from build123d import *

# Parameters (mm, degrees)
SKETCH1_R                 = 3.2639
BOSS_EXTRUDE1_DEPTH       = 12.7
SKETCH2_W                 = 12.7
SKETCH2_H                 = 12.7
CUT_EXTRUDE1_DEPTH        = 6.35
SKETCH3_W                 = 9.525
SKETCH3_H                 = 12.7
CUT_EXTRUDE2_DEPTH        = 9.525
F_6_32_TAPPED_HOLE1_D     = 2.7051
F_6_32_TAPPED_HOLE1_DEPTH = 15.875
F_6_32_TAPPED_HOLE1_TIP   = 0.81269403


with BuildPart() as part:
    # Sketch1 → Boss-Extrude1 (new body)
    with BuildSketch(Plane.XY):
        with BuildLine():
            Line((-7.9375, 13.335), (-7.9375, 38.1))
            Line((-7.9375, 38.1), (7.9375, 38.1))
            Line((7.9375, 38.1), (7.9375, 13.335))
            ThreePointArc((7.9375, 13.335), (9.983359133, 8.395859133), (14.9225, 6.35))
            Line((14.9225, 6.35), (66.294, 6.35))
            ThreePointArc((66.294, 6.35), (66.563407684, 6.238407684), (66.675, 5.969))
            Line((66.675, 5.969), (66.675, -5.969))
            ThreePointArc((66.675, -5.969), (66.563407684, -6.238407684), (66.294, -6.35))
            Line((66.294, -6.35), (-66.294, -6.35))
            ThreePointArc((-66.294, -6.35), (-66.563407684, -6.238407684), (-66.675, -5.969))
            Line((-66.675, -5.969), (-66.675, 5.969))
            ThreePointArc((-66.675, 5.969), (-66.563407684, 6.238407684), (-66.294, 6.35))
            Line((-66.294, 6.35), (-14.9225, 6.35))
            ThreePointArc((-14.9225, 6.35), (-9.983359133, 8.395859133), (-7.9375, 13.335))
        make_face()
        with Locations((-60.325, 0)):
            Circle(SKETCH1_R, mode=Mode.SUBTRACT)
        with Locations((60.325, 0)):
            Circle(SKETCH1_R, mode=Mode.SUBTRACT)
    extrude(amount=BOSS_EXTRUDE1_DEPTH)

    # Sketch2 → Cut-Extrude1 (cut)
    with BuildSketch(Plane(origin=(0, 0, 0), x_dir=(-1, 0, 0), z_dir=(0, 0, -1))):
        with Locations((-60.325, 0)):
            Rectangle(SKETCH2_W, SKETCH2_H)
        with Locations((60.325, 0)):
            Rectangle(SKETCH2_W, SKETCH2_H)
    extrude(amount=-CUT_EXTRUDE1_DEPTH, mode=Mode.SUBTRACT)

    # Sketch3 → Cut-Extrude2 (cut)
    with BuildSketch(Plane(origin=(0, 38.1, 0), x_dir=(1, 0, 0), z_dir=(0, 1, 0))):
        with Locations((0, -6.35)):
            Rectangle(SKETCH3_W, SKETCH3_H)
    extrude(amount=-CUT_EXTRUDE2_DEPTH, mode=Mode.SUBTRACT)

    # #6-32 Tapped Hole1
    with Locations(Plane(origin=(0, 28.575, 0), x_dir=(1, 0, 0), z_dir=(0, 1, 0))):
        with Locations((0, -3.175), (0, -9.525)):
            Hole(F_6_32_TAPPED_HOLE1_D / 2, depth=F_6_32_TAPPED_HOLE1_DEPTH)
            with Locations((0, 0, -(F_6_32_TAPPED_HOLE1_DEPTH + F_6_32_TAPPED_HOLE1_TIP / 2))):  # 118° drill point
                Cone(0, F_6_32_TAPPED_HOLE1_D / 2, F_6_32_TAPPED_HOLE1_TIP, mode=Mode.SUBTRACT)


solid = part.part
Verification items for the finished model (mm, model axes). A direction names the side the tool comes from. Give positions to 0.01 mm unless a question says otherwise; leave off trailing zeros. Write each loop counter-clockwise with the first axis right and the second up, starting at its lowest first coordinate (ties: lowest second). Pieces come first, ordered by that corner, then holes. Notation, with made-up numbers: M 84.25,6 L 114.25,6 A24 cw 114.25,25 Z; hole C 71.5,51.5 d11. An arc over 180 degrees is marked long. Write item = value, one per line.
(1) Draft check along X on faces 1 (the face through (-4.762, 33, 6)), 2 (the face through (-53.975, 0, 3)), 3 (the face through (9.93, 8.45, 6.26)). Enter one of: released by +X, released by -X, zero draft, split by the parting line, or undercut.
Found:
face_1 = undercut
face_2 = released by -X
face_3 = released by +X
(2) Sectioned sample at C-C (x = 3.5). Record the cut outline in (y, z) (3 decimals), then the cut area to 3 significant figures.
Found:
outline = M -6.35,0 L 28.575,0 L 28.575,12.7 L -6.35,12.7 Z
area = 444 mm2
(3) Access from +Z, -Z, +X, -X, +Y, -Y to the whole of each face (thin tool, end or side, straight path). Record for faces 4 (the face through (40, 6.35, 6)), 5 (the face through (62, 3, 6.35)), 6 (the face through (0, 28.575, 6)).
Found:
face_4 = +Z, -Z, +X, +Y
face_5 = -Z, +X, +Y, -Y
face_6 = +Z, -Z, +Y
(4) Go/stop test with flat-tipped pins: pin 1 Ø1.6 at (x, z) = (0, 9.525) entering from +Y; pin 2 Ø3 at (x, z) = (-2, 7.5) entering from +Y (3 decimals); pin 3 Ø4 at (x, z) = (28.5, 7) entering from +Y; pin 4 Ø7 at (y, z) = (-3, 4) entering from +X (3 decimals). Record where each tip stops, or that it passes through.
Found:
pin_1 = 12.37
pin_2 = 28.575
pin_3 = 6.35
pin_4 = 66.675
(5) Sectioned sample at B-B (x = 25). Record the cut outline in (y, z).
Found:
outline = M -6.35,0 L 6.35,0 L 6.35,12.7 L -6.35,12.7 Z
(6) Material ranges on line 1 (Z direction, x = 0, y = 22); line 2 (X direction, y = 0, z = 11.5) (3 decimals); line 3 (X direction, y = 2, z = 8.25) (3 decimals), recorded low to high.
Found:
line_1 = 0 to 1.82, 4.53 to 8.17, 10.88 to 12.7
line_2 = -66.675 to -63.589, -57.061 to 57.061, 63.589 to 66.675
line_3 = -66.675 to -62.904, -57.746 to 57.746, 62.904 to 66.675
(7) Sectioned sample at A-A (y = 0). Record the cut outline in (x, z) (3 decimals), then the cut area to 3 significant figures.
Found:
outline = M -66.675,6.35 L -63.589,6.35 L -63.589,12.7 L -66.675,12.7 Z; M -57.061,6.35 L -53.975,6.35 L -53.975,0 L 53.975,0 L 53.975,6.35 L 57.061,6.35 L 57.061,12.7 L -57.061,12.7 Z; M 63.589,6.35 L 66.675,6.35 L 66.675,12.7 L 63.589,12.7 Z
area = 1,450 mm2
